CAD build for the part. Positions are in the model's coordinates, mm. A direction names the side the tool comes from. Give positions to 0.01 mm unless a question says otherwise; leave off trailing zeros. Order: outer loops, then holes, each group sorted by start corner. A loop starts at its lowest first (then second) coordinate and runs counter-clockwise, first axis right, second up. Notation, with made-up numbers: M -4,-7.5 L 4,-7.5 A15 ccw 4,3.5 Z; hole C 53,-10.5 d11. An arc over 180 degrees is marked long. Put each result on its own line as item: value. Start each with the question number.
1) Cut at A-A (x = -12.7). Write the cut outline in (y, z), and give its area (3 significant figures).
2) Cut at C-C (y = 12.7). Write the cut outline in (x, z) (3 decimals), and give its area (3 significant figures).
3) Tool access for faces 4 (the face through (-3.175, 25, -14)), 5 (the face through (-1.565, 14.752, -12.431)): list every direction of +Z, -Z, +X, -X, +Y, -Y with a clear straight run to the whole face (end or side of a thin tool).
4) Cut at D-D (y = 4). Write the cut outline in (x, z) (3 decimals).
5) Two-plate mould, pull along Z, no slides. Class faces 1 (the face through (-1.57, 36.08, -12.25)), 2 (the face through (0, 25, -13)), 3 (the face through (-14, 25, -3.048)): released by +Z, released by -Z, zero draft, split by the parting line, or undercut.
6) Cut at B-B (z = -12.7). Write the cut outline in (x, y) (3 decimals).
7) Drill centre lines: line 1 (Y direction, x = -2.3, z = -12.7); line 2 (Z direction, x = -6.75, y = 38.5); line 3 (X direction, y = 37, z = -10.75) (3 decimals). Where is each one in solid material? Low to high. Write a range as [from, to].
8) Pin check, flat tips, straight feed: pin 1 (12 mm diameter, centred on y = 10.5, z = -15, fed in from -X) (3 decimals); pin 2 (11 mm diameter, centred on x = -18.5, y = 26, fed in from -Z). Stop position of each tip, or through.
Autodesk Inventor part; units mm, degrees
ref_plane "YZ Plane" through (0, 0, 0) normal (1, 0, 0) x (0, 1, 0)
ref_plane "XZ Plane" through (0, 0, 0) normal (0, 1, 0) x (-1, 0, 0)
ref_plane "XY Plane" through (0, 0, 0) normal (0, 0, 1) x (1, 0, 0)
sketch "Sketch1" plane through (0, 0, 0) normal (0, 1, 0) x (-1, 0, 0)
  line L0 (0, 0) -> (0, -25.4)
  line L1 (0, -25.4) -> (0, 0)
  line L2 (0, 0) -> (25.4, 0)
  line L3 (25.4, 0) -> (25.4, -3.048)
  line L4 (25.4, -3.048) -> (3.175, -3.048)
  line L5 (3.175, -3.048) -> (3.175, -25.4)
  line L6 (3.175, -25.4) -> (0, -25.4)
  dimension "d0" = 25.4
  dimension "d1" = 25.4
  dimension "d2" = 3.048
  dimension "d3" = 3.175
extrude "Extrusion1" add sketch "Sketch1" along normal blind 50.8
sketch "Sketch2" plane through (-25.4, 0, 0) normal (0, 0, 1) x (1, 0, 0)
  line L0 (22.225, 50.8) -> (0, 50.8) construction
  line L1 (22.225, 0) -> (0, 0) construction
  line L2 (12.7, 50.8) -> (12.7, 0) construction
  line L3 (0, 0) -> (0, 50.8) construction
  circle A0 centre (12.7, 12.7) radius 2.0701
  circle A1 centre (12.7, 38.1) radius 2.0701
  line L4 (25.4, 0) -> (25.4, 50.8)
  dimension "d7" = 4.1402
  dimension "d8" = 4.1402
  dimension "d9" = 25.4
  dimension "d10" = 12.7
  dimension "d16" = 12.7
sketch "Sketch3" plane through (0, 0, 0) normal (1, 0, 0) x (0, 0, -1)
  line L0 (0, 0) -> (25.4, 0)
  line L1 (25.4, 0) -> (25.4, 50.8)
  line L2 (0, 50.8) -> (25.4, 50.8)
  line L3 (0, 0) -> (0, 50.8)
  circle A0 centre (12.7, 38.1) radius 2.0701
  circle A1 centre (12.7, 12.7) radius 2.0701
  dimension "d11" = 4.1402
  dimension "d12" = 4.1402
  dimension "d13" = 12.7
  dimension "d14" = 12.7
  dimension "d15" = 25.4
extrude "Extrusion2" cut sketch "Sketch2" against normal through all
extrude "Extrusion3" cut sketch "Sketch3" against normal blind 25.4 contours A0 | A1
properties part number "LBracketConnectors"
Solution:
1. outline: M 0,-3.05 L 10.63,-3.05 L 10.63,0 L 0,0 Z; M 14.77,-3.05 L 36.03,-3.05 L 36.03,0 L 14.77,0 Z; M 40.17,-3.05 L 50.8,-3.05 L 50.8,0 L 40.17,0 Z
1. area: 130 mm²
2. outline: M -25.4,-3.048 L -14.77,-3.048 L -14.77,0 L -25.4,0 Z; M -10.63,-3.048 L -3.175,-3.048 L -3.175,-10.63 L 0,-10.63 L 0,0 L -10.63,0 Z; M -3.175,-25.4 L 0,-25.4 L 0,-14.77 L -3.175,-14.77 Z
2. area: 123 mm²
3. face 4: -Z, -X, +Y, -Y
3. face 5: +X, -X
4. outline: M -25.4,-3.048 L -3.175,-3.048 L -3.175,-25.4 L 0,-25.4 L 0,0 L -25.4,0 Z
5. face 1: undercut
5. face 2: zero draft
5. face 3: released by -Z
6. outline: M -3.175,0 L 0,0 L 0,10.63 L -3.175,10.63 Z; M -3.175,14.77 L 0,14.77 L 0,36.03 L -3.175,36.03 Z; M -3.175,40.17 L 0,40.17 L 0,50.8 L -3.175,50.8 Z
7. line 1: [0, 10.63], [14.77, 36.03], [40.17, 50.8]
7. line 2: [-3.05, 0]
7. line 3: [-3.175, 0]
8. pin 1: x = -3.175
8. pin 2: z = -3.05
